from build123d import *

# Parameters (mm, degrees)
SKETCH_1_W      = 90
SKETCH_1_H      = 65
SKETCH_1_W_2    = 10
SKETCH_1_H_2    = 3
SKETCH_1_W_3    = 3
SKETCH_1_H_3    = 10
EXTRUDE_1_DEPTH = 3


with BuildPart() as part:
    # 草图1 → 凸台-拉伸1 (new body)
    with BuildSketch(Plane.XY):
        Rectangle(SKETCH_1_W, SKETCH_1_H)
        with Locations((-10, 29)):
            Rectangle(SKETCH_1_W_2, SKETCH_1_H_2, mode=Mode.SUBTRACT)
        with Locations((-30, 29)):
            Rectangle(SKETCH_1_W_2, SKETCH_1_H_2, mode=Mode.SUBTRACT)
        with Locations((-41.5, 20)):
            Rectangle(SKETCH_1_W_3, SKETCH_1_H_3, mode=Mode.SUBTRACT)
        with Locations((10, 29)):
            Rectangle(SKETCH_1_W_2, SKETCH_1_H_2, mode=Mode.SUBTRACT)
        with Locations((30, 29)):
            Rectangle(SKETCH_1_W_2, SKETCH_1_H_2, mode=Mode.SUBTRACT)
        with Locations((-41.5, 0)):
            Rectangle(SKETCH_1_W_3, SKETCH_1_H_3, mode=Mode.SUBTRACT)
        with Locations((-41.5, -20)):
            Rectangle(SKETCH_1_W_3, SKETCH_1_H_3, mode=Mode.SUBTRACT)
        with Locations((41.5, -20)):
            Rectangle(SKETCH_1_W_3, SKETCH_1_H_3, mode=Mode.SUBTRACT)
        with Locations((41.5, 0)):
            Rectangle(SKETCH_1_W_3, SKETCH_1_H_3, mode=Mode.SUBTRACT)
        with Locations((41.5, 20)):
            Rectangle(SKETCH_1_W_3, SKETCH_1_H_3, mode=Mode.SUBTRACT)
        with Locations((30, -29)):
            Rectangle(SKETCH_1_W_2, SKETCH_1_H_2, mode=Mode.SUBTRACT)
        with Locations((10, -29)):
            Rectangle(SKETCH_1_W_2, SKETCH_1_H_2, mode=Mode.SUBTRACT)
        with Locations((-10, -29)):
            Rectangle(SKETCH_1_W_2, SKETCH_1_H_2, mode=Mode.SUBTRACT)
        with Locations((-30, -29)):
            Rectangle(SKETCH_1_W_2, SKETCH_1_H_2, mode=Mode.SUBTRACT)
    extrude(amount=EXTRUDE_1_DEPTH)


solid = part.part
Here's how the part is built. I have some questions about the finished solid (model axes, mm). Coordinates: 2 decimals unless noted, no trailing zeros. Write each loop counter-clockwise with the first axis right and the second up, starting at its lowest first coordinate (ties: lowest second). Pieces come first, ordered by that corner, then holes.
Item 1: I want a section at A-A on x = -13. Write out the boundary of the cut face in (y, z), and give its area (3 significant figures).
Item 2: I want a section at B-B on y = -24. Write out the boundary of the cut face in (x, z).
Item 3: I want a section at C-C on z = 2.5. Count the separate pieces of the cut face and the enclosed holes in it, and give its area (3 significant figures).
Item 4: If we mould it in two halves opening along Y, with no side actions, what happens to faces 1 (the flat face through (35, -29, 1)), 2 (the flat face through (-1, 0, 3))? For each: +Y half, -Y half, draft (parallel to the pull), parting line (faces both ways), or undercut.
Item 5: If I drill on line 1 (Y direction, x = 41, z = 2.8); line 2 (X direction, y = 4.5, z = 2.1); line 3 (Y direction, x = -29.5, z = 0.5), over which ranges is the centre line in solid material (lowest first)?
Findings below:
1. outline: (-32.5, 0) - (-30.5, 0) - (-30.5, 3) - (-32.5, 3) - close; (-27.5, 0) - (27.5, 0) - (27.5, 3) - (-27.5, 3) - close; (30.5, 0) - (32.5, 0) - (32.5, 3) - (30.5, 3) - close
1. area: 177 mm2
2. outline: (-45, 0) - (-43, 0) - (-43, 3) - (-45, 3) - close; (-40, 0) - (40, 0) - (40, 3) - (-40, 3) - close; (43, 0) - (45, 0) - (45, 3) - (43, 3) - close
3. separate pieces: 1
3. enclosed holes: 14
3. area: 5,430 mm2
4. face 1: undercut
4. face 2: draft
5. line 1: y = -32.5 to -25, -15 to -5, 5 to 15, 25 to 32.5
5. line 2: x = -45 to -43, -40 to 40, 43 to 45
5. line 3: y = -32.5 to -30.5, -27.5 to 27.5, 30.5 to 32.5
